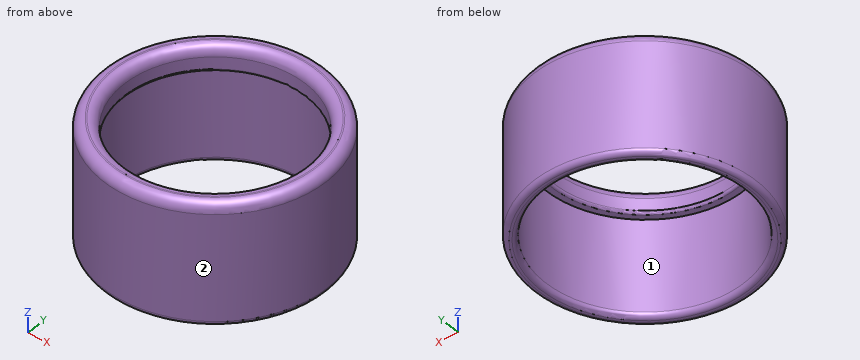
Autodesk Inventor part; units mm, degrees
ref_plane "YZ Plane" through (0, 0, 0) normal (1, 0, 0) x (0, 1, 0)
ref_plane "XZ Plane" through (0, 0, 0) normal (0, 1, 0) x (-1, 0, 0)
ref_plane "XY Plane" through (0, 0, 0) normal (0, 0, 1) x (1, 0, 0)
sketch "Sketch1" plane through (0, 0, 0) normal (0, 0, 1) x (1, 0, 0)
  point P0 (0, 0)
sketch "Sketch2" plane through (0, 0, 0) normal (0, 0, 1) x (1, 0, 0)
  circle A0 centre (0, 0) radius 18.8587
  circle A1 centre (0, 0) radius 20.6375
  dimension "d0" = 37.7174
  dimension "d1" = 41.275
extrude "Extrusion1" add sketch "Sketch2" along normal blind 5
sketch "Sketch3" plane through (0, 0, 0) normal (0, 0, -1) x (-1, 0, 0)
  circle A0 centre (0, 0) radius 20.6375
  circle A1 centre (0, 0) radius 23.1375
  dimension "d4" = 46.275
extrude "Extrusion2" add sketch "Sketch3" along normal blind 20 and the other way blind 5
fillet "Fillet5" radius 1 2 edges at (20.6375, 0, -20) (23.1375, 0, -20)
fillet "Fillet6" radius 2 2 edges at (-18.8587, 0, 5) (23.1375, 0, 5)
fillet "Fillet7" radius 0.5 1 edges at (-18.8587, 0, 0)
properties part number "5200_Biax_TxRx_Relative_Position_AirFlowGuide_MPSv2_v3" material "Acetal Resin, White"
Could you check a few things on this model? Use its own coordinates, in mm. Face numbers are marked on the shaded views. Coordinates: 2 decimals unless noted, no trailing zeros. Write each loop counter-clockwise with the first axis right and the second up, starting at its lowest first coordinate (ties: lowest second). Pieces come first, ordered by that corner, then holes. Notation, with made-up numbers: (11, 18) -> (16, 18) arc R21 ccw to (16, 24) -> close; hole circle Ø6 at (-17.75, 78.25). An arc over 180 degrees is marked (long way). Write item = value, one per line. Start each with the question number.
(1) I want a section at A-A (x = 0). Please give me the cut outline in (y, z), plus the area to 3 significant figures.
(2) Will these pins go through, and if not, where does the flat tip stop? pin 1 (10 mm diameter, centred on x = 2.5, y = 14, fed in from +Z); pin 2 (12 mm diameter, centred on x = 7.5, z = -6.5, fed in from +Y); pin 3 (2 mm diameter, centred on x = 15, z = -7, fed in from +Y).
(3) We'd pull the mould along Y, two halves only. Please class the marked faces 1 and 2: released by +Y, released by -Y, zero draft, split by the parting line, or undercut.
(4) I need wall thicknesses on line 1 (Y direction, x = 0, z = -4.75); line 2 (Z direction, x = 12.5, y = -16.5); line 3 (Y direction, x = 0, z = 1.75). Which ranges of each line are inside material? Lowest first, please. Write a range as [from, to].
Result set:
q1.outline = (-23.14, -19) arc R1 ccw to (-22.14, -20) -> (-21.64, -20) arc R1 ccw to (-20.64, -19) -> (-20.64, 0) -> (-19.36, 0) arc R0.5 ccw to (-18.86, 0.5) -> (-18.86, 3) arc R2 ccw to (-20.86, 5) -> (-21.14, 5) arc R2 ccw to (-23.14, 3) -> close; (18.86, 0.5) arc R0.5 ccw to (19.36, 0) -> (20.64, 0) -> (20.64, -19) arc R1 ccw to (21.64, -20) -> (22.14, -20) arc R1 ccw to (23.14, -19) -> (23.14, 3) arc R2 ccw to (21.14, 5) -> (20.86, 5) arc R2 ccw to (18.86, 3) -> close
q1.area = 138 mm2
q2.pin_1 = 4.15
q2.pin_2 = 23.09
q2.pin_3 = 18.42
q3.face_1 = undercut
q3.face_2 = split by the parting line
q4.line_1 = [-23.14, -20.64], [20.64, 23.14]
q4.line_2 = [-19.35, 4.99]
q4.line_3 = [-23.14, -18.86], [18.86, 23.14]
